For this review, take the finished solid that the model builds, in its own axes (mm). Face numbers are marked on the shaded views. A direction names the side the tool comes from. Give positions to 0.01 mm unless a question says otherwise; leave off trailing zeros. Write each loop counter-clockwise with the first axis right and the second up, starting at its lowest first coordinate (ties: lowest second). Pieces come first, ordered by that corner, then holes. Notation, with made-up numbers: M 45,55 L 81,55 A11 ccw 81,73 Z; hole C 20,-30 d2. An arc over 180 degrees is marked long. Write item = value, one per line.
```python
from build123d import *
from build123d.topology import SkipClean

# Parameters (mm, degrees)
SKETCH9_R          = 4
SKETCH9_R_2        = 3.238
EXTRUDE1_DEPTH     = 5.0625
REVOLVE2_ANGLE     = 90
EXTRUDE2_DEPTH     = 5.25
EXTRUDE5_START     = -5.25
SKETCH16_R         = 5.0625
SKETCH16_R_2       = 3.238
EXTRUDE5_DEPTH     = 5.25
SKETCH12_R         = 3.238
CUT_EXTRUDE1_DEPTH = 25.90230913
CUT_EXTRUDE2_START = 5.0625
SKETCH13_R         = 3.238
CUT_EXTRUDE2_DEPTH = 5.0625
SKETCH15_R         = 4
SKETCH15_R_2       = 3.238
EXTRUDE4_DEPTH     = 21.5
CHAMFER1_SIZE      = 0.381


with BuildPart() as part:
    # Sketch8 → Revolve1 (revolve)
    with BuildSketch(Plane(origin=(0, 0, 0), x_dir=(0, 0, -1), z_dir=(1, 0, 0)), mode=Mode.PRIVATE) as revolve1_sk:
        with BuildLine():
            Line((21.603, 6.075), (22.238, 6.075))
            ThreePointArc((22.238, 6.075), (22.776815367, 5.851815367), (23, 5.313))
            Line((23, 5.313), (23, 4.381))
            Line((23, 4.381), (22.619, 4))
            Line((22.619, 4), (0, 4))
            Line((0, 4), (0, 5.0625))
            Line((0, 5.0625), (8.05, 5.0625))
            Line((8.05, 5.0625), (10.972835738, 6.75))
            Line((10.972835738, 6.75), (20.587, 6.75))
            Line((20.587, 6.75), (20.587, 5.4675))
            Line((20.587, 5.4675), (21.603, 5.4675))
            Line((21.603, 5.4675), (21.603, 6.075))
        make_face()
    revolve(revolve1_sk.sketch.rotate(Axis((0, 0, 0), (0, 0, -1)), 90), axis=Axis((0, 0, 0), (0, 0, -1)))

    # Sketch9 → Extrude1 (add)
    with BuildSketch(Plane.XY):
        Circle(SKETCH9_R)
        Circle(SKETCH9_R_2, mode=Mode.SUBTRACT)
    extrude(amount=-EXTRUDE1_DEPTH)

    # Sketch11 → Revolve2 (revolve)
    with BuildSketch(Plane.XY):
        with BuildLine():
            Line((-5.0625, 0), (-3.238, 0))
            ThreePointArc((-3.238, 0), (0, -3.238), (3.238, 0))
            Line((3.238, 0), (5.0625, 0))
            ThreePointArc((5.0625, 0), (0, -5.0625), (-5.0625, 0))
        make_face()
    revolve(axis=Axis((-5.0625, 0, 0), (-1, 0, 0)), revolution_arc=REVOLVE2_ANGLE)

    # Sketch14 → Extrude2 (add)
    with BuildSketch(Plane(origin=(0, 0, 0), x_dir=(-1, 0, 0), z_dir=(0, 1, 0))):
        with BuildLine():
            Line((-5.0625, 0), (-3.238, 0))
            ThreePointArc((-3.238, 0), (0, 3.238), (3.238, 0))
            Line((3.238, 0), (5.0625, 0))
            ThreePointArc((5.0625, 0), (0, 5.0625), (-5.0625, 0))
        make_face()
    extrude(amount=EXTRUDE2_DEPTH)

    # Sketch16 → Extrude5 (add)
    with SkipClean():  # the faces are left unmerged after this step: merging them gives an invalid solid
        with BuildSketch(Plane(origin=(0, 5.25, 0), x_dir=(-1, 0, 0), z_dir=(0, 1, 0)).offset(EXTRUDE5_START)):
            with Locations(Location((0, 0, 0), (0, 0, 180))):
                Circle(SKETCH16_R)
            with Locations(Location((0, 0, 0), (0, 0, 180))):
                Circle(SKETCH16_R_2, mode=Mode.SUBTRACT)
        extrude(amount=EXTRUDE5_DEPTH)

    # Sketch12 → Cut-Extrude1 (cut, through all)
    with BuildSketch(Plane(origin=(0, 0, 0), x_dir=(1, 0, 0), z_dir=(0, 1, 0))):
        Circle(SKETCH12_R)
    extrude(amount=CUT_EXTRUDE1_DEPTH, mode=Mode.SUBTRACT)

    # Sketch13 → Cut-Extrude2 (cut)
    with BuildSketch(Plane.XY.offset(-5.0625).offset(CUT_EXTRUDE2_START)):
        Circle(SKETCH13_R)
    extrude(amount=-CUT_EXTRUDE2_DEPTH, mode=Mode.SUBTRACT)

    # Sketch15 → Extrude4 (add)
    with BuildSketch(Plane(origin=(0, 5.25, 0), x_dir=(-1, 0, 0), z_dir=(0, 1, 0))):
        with Locations(Location((0, 0, 0), (0, 0, 90))):
            Circle(SKETCH15_R)
        with Locations(Location((0, 0, 0), (0, 0, 180))):
            Circle(SKETCH15_R_2, mode=Mode.SUBTRACT)
    extrude(amount=EXTRUDE4_DEPTH)

    # Chamfer1
    chamfer1_edges = [part.edges().sort_by_distance(p)[0] for p in [
        (0, 26.75, -4),
    ]]
    chamfer(chamfer1_edges, length=CHAMFER1_SIZE)


solid = part.part
```
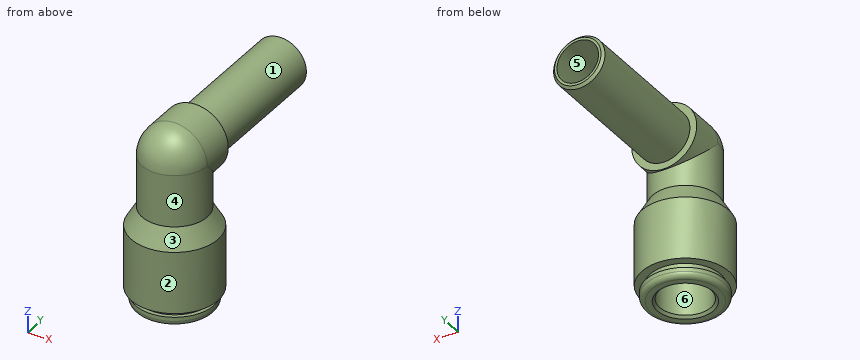
1. We need section B-B, the plane z = -17. Write out the cut boundary in (x, y), then the cut area to 3 significant figures.
Responses:
outline = C 0,0 d13.5; hole C 0,0 d8
area = 92.9 mm2
2. Insertion check: P1, Ø5, axis at x = -2.5, y = 21, coming from the -Z side; P2, Ø7, axis at x = 0, y = 0, coming from the -Z side; P3, Ø1, axis at x = -1.5, y = 22, coming from the +Z side; P4, Ø3, axis at x = 1.5, z = -2.5, coming from the +Y side. Each pin has a flat end and moves straight along its axis. Give the tip position at first contact, or say it passes through.
Responses:
P1 = -4
P2 = -5.06
P3 = 3.87
P4 = 26.75
3. For line 1 along Y through (x, z) = (0, -16); line 2 along Y through (x, z) = (1.5, -6); line 3 along X through (y, z) = (3.5, -20.25), list the stretches that pass through material, from the lowest coordinate up. Write a range as from..to.
Responses:
line_1 = -6.75..-4, 4..6.75
line_2 = -4.84..-3.71, 3.71..4.84
line_3 = -5.77..-1.94, 1.94..5.77
4. We need section A-A, the plane y = 8. Write out the cut boundary in (x, z), then the cut area to 3 significant figures.
Responses:
outline = C 0,0 d8; hole C 0,0 d6.48
area = 17.3 mm2
5. The part is to be moulded in two halves that separate along Y. For the marked faces 4, 5 and 6, say which applies: +Y half, -Y half, draft (parallel to the pull), parting line (faces both ways), or undercut.
Responses:
face_4 = parting line
face_5 = draft
face_6 = undercut
6. Machinability: for the marked faces 1, 2 and 3, which of the approach directions +Z, -Z, +X, -X, +Y, -Y give a long, thin tool a straight path to every point of the face, cutting with its end or side? Answer none if there is none.
Responses:
face_1 = +Y
face_2 = -Z
face_3 = none
